For this review, take the finished solid that the model builds, in its own axes (mm). A direction names the side the tool comes from. Coordinates: 2 decimals unless noted, no trailing zeros. Write each loop counter-clockwise with the first axis right and the second up, starting at its lowest first coordinate (ties: lowest second). Pieces come first, ordered by that corner, then holes.
1) Insertion check: P1, Ø8, axis at x = 144, y = 25, coming from the -Z side; P2, Ø6, axis at x = -24, z = -267.5, coming from the +Y side; P3, Ø19, axis at x = 341.5, z = -163.5, coming from the +Y side. Each pin has a flat end and moves straight along its axis. Give the tip position at first contact, or say it passes through.
2) For faces 5 (the face through (-365.125, 2, -288)), 6 (the face through (327.025, -145, -235)), 7 (the face through (-327.025, 140, -235)), 8 (the face through (346, 139.7, -151)), 9 (the face through (-5, 139.7, -19)), list the 3-axis set-ups (+Z, -Z, +X, -X, +Y, -Y) from which the entire face can be reached by the end or side of a thin tool; tool diameter is ignored.
3) We need section A-A on y = 4.5. Write out the cut boundary in (x, z) (3 decimals), then the cut area to 3 significant figures.
4) Mouldability with a two-part tool opening along Z and no side actions: class faces 1 (the face through (-346, -139.7, -151)), 2 (the face through (346, 158, -342.9)), 3 (the face through (-346, -2, -38.1)), 4 (the face through (-5, 19.05, -286)) as pulls with the +Z half, pulls with the -Z half, needs draft (parallel to the pull), parting line crosses it, or undercut.
5) We need section D-D on x = 157. Write out the cut boundary in (y, z).
6) We need section C-C on z = -81.5. Write out the cut boundary in (x, y) (3 decimals).
7) To check wall thickness, follow line 1 along X through (y, z) = (-23.5, -14.5) (3 decimals); line 2 along Z through (x, y) = (68, -15); line 3 along Z through (x, y) = (328.5, -10.5). State the ranges of each line that lie inside material, in increasing order.
8) We need section B-B on y = 114.5. Write out the cut boundary in (x, z) (3 decimals).
from build123d import *

# Parameters (mm, degrees)
F0_W      = 755.65
F0_H      = 381
F1_DEPTH  = 38.1
F2_W      = 730.25
F2_H      = 355.6
F2_W_2    = 654.05
F2_H_2    = 279.4
F3_DEPTH  = 38.1
F4_W      = 38.1
F4_H      = 38.1
F5_DEPTH  = 304.8
F6_W      = 355.6
F6_H      = 38.1
F7_DEPTH  = 38.1
F8_W      = 355.6
F8_H      = 38.1
F9_DEPTH  = 38.1
F10_W     = 730.25
F10_H     = 38.1
F11_DEPTH = 38.1


with BuildPart() as f1:
    # F0 (on Top) → F1 (new body)
    with BuildSketch(Plane.XY):
        Rectangle(F0_W, F0_H)
    extrude(amount=F1_DEPTH)

    # F2 (on face) → F3 (join)
    with BuildSketch(Plane(origin=(0, 0, 0), x_dir=(1, 0, 0), z_dir=(0, 0, -1))):
        Rectangle(F2_W, F2_H)
        Rectangle(F2_W_2, F2_H_2, mode=Mode.SUBTRACT)
    extrude(amount=F3_DEPTH)

    # F4 (on face) → F5 (join)
    with BuildSketch(Plane(origin=(0, 0, -38.1), x_dir=(1, 0, 0), z_dir=(0, 0, -1))):
        with Locations((-346.075, 158.75)):
            Rectangle(F4_W, F4_H)
        with Locations((346.075, 158.75)):
            Rectangle(F4_W, F4_H)
        with Locations((346.075, -158.75)):
            Rectangle(F4_W, F4_H)
        with Locations((-346.075, -158.75)):
            Rectangle(F4_W, F4_H)
    extrude(amount=F5_DEPTH)

    # F6 (on face) → F7 (join)
    with BuildSketch(Plane(origin=(-365.125, 0, 0), x_dir=(0, -1, 0), z_dir=(-1, 0, 0))):
        with Locations((0, -285.75)):
            Rectangle(F6_W, F6_H)
    extrude(amount=-F7_DEPTH)

    # F8 (on face) → F9 (join)
    with BuildSketch(Plane.YZ.offset(365.125)):
        with Locations((0, -285.75)):
            Rectangle(F8_W, F8_H)
    extrude(amount=-F9_DEPTH)

    # F10 (on face) → F11 (join)
    with BuildSketch(Plane(origin=(0, 0, -304.8), x_dir=(1, 0, 0), z_dir=(0, 0, -1))):
        Rectangle(F10_W, F10_H)
    extrude(amount=-F11_DEPTH)


solid = f1.part
Result:
1. P1: stops at z = 0
1. P2: stops at y = 19.05
1. P3: stops at y = 177.8
2. face 5: -Z, -X, +Y, -Y
2. face 6: -Z, -Y
2. face 7: -Z, +Y
2. face 8: +X, -X
2. face 9: -Z
3. outline: (-377.825, 0) - (-365.125, 0) - (-365.125, -38.1) - (-327.025, -38.1) - (-327.025, 0) - (327.025, 0) - (327.025, -38.1) - (365.125, -38.1) - (365.125, 0) - (377.825, 0) - (377.825, 38.1) - (-377.825, 38.1) - close; (-365.125, -304.8) - (365.125, -304.8) - (365.125, -266.7) - (-365.125, -266.7) - close
3. area: 59,500 mm2
4. face 1: undercut
4. face 2: pulls with the -Z half
4. face 3: undercut
4. face 4: needs draft
5. outline: (-190.5, 0) - (-177.8, 0) - (-177.8, -38.1) - (-139.7, -38.1) - (-139.7, 0) - (139.7, 0) - (139.7, -38.1) - (177.8, -38.1) - (177.8, 0) - (190.5, 0) - (190.5, 38.1) - (-190.5, 38.1) - close; (-19.05, -304.8) - (19.05, -304.8) - (19.05, -266.7) - (-19.05, -266.7) - close
6. outline: (-365.125, -177.8) - (-327.025, -177.8) - (-327.025, -139.7) - (-365.125, -139.7) - close; (-365.125, 139.7) - (-327.025, 139.7) - (-327.025, 177.8) - (-365.125, 177.8) - close; (327.025, -177.8) - (365.125, -177.8) - (365.125, -139.7) - (327.025, -139.7) - close; (327.025, 139.7) - (365.125, 139.7) - (365.125, 177.8) - (327.025, 177.8) - close
7. line 1: x = -365.125 to -327.025, 327.025 to 365.125
7. line 2: z = -304.8 to -266.7, 0 to 38.1
7. line 3: z = -304.8 to -266.7, -38.1 to 38.1
8. outline: (-377.825, 0) - (-365.125, 0) - (-365.125, -38.1) - (-327.025, -38.1) - (-327.025, 0) - (327.025, 0) - (327.025, -38.1) - (365.125, -38.1) - (365.125, 0) - (377.825, 0) - (377.825, 38.1) - (-377.825, 38.1) - close; (-365.125, -304.8) - (-327.025, -304.8) - (-327.025, -266.7) - (-365.125, -266.7) - close; (327.025, -304.8) - (365.125, -304.8) - (365.125, -266.7) - (327.025, -266.7) - close
